Geometry check sheet. Reference: the model listing, model coordinates, mm. A direction names the side the tool comes from. Coordinates: 2 decimals unless noted, no trailing zeros. Loops run counter-clockwise (first coordinate to the right, second up) from the corner with the lowest first, then second, coordinate; pieces in that order, holes last.
from build123d import *
from build123d.topology import SkipClean

# Parameters (mm, degrees)
BOSS_EXTRUDE1_DEPTH = 10
BOSS_EXTRUDE2_DEPTH = 7.5
BOSS_EXTRUDE3_DEPTH = 5


with BuildPart() as part:
    # Sketch1 → Boss-Extrude1 (new, symmetric)
    with SkipClean():  # the faces are left unmerged after this step: merging them gives an invalid solid
        with BuildSketch(Plane.XY):
            with BuildLine():
                Line((-10, 54.083269132), (-10, 42.848570571))
                ThreePointArc((-10, 42.848570571), (0, 44), (10, 42.848570571))
                Line((10, 42.848570571), (10, 54.083269132))
                Line((10, 54.083269132), (10, 89))
                Line((10, 89), (10, 95.679491924))
                ThreePointArc((10, 95.679491924), (0, 93), (-10, 95.679491924))
                Line((-10, 95.679491924), (-10, 89))
                Line((-10, 89), (-10, 54.083269132))
            make_face()
            with BuildLine():
                ThreePointArc((-42.848570571, -10), (-44, 0), (-42.848570571, 10))
                Line((-42.848570571, 10), (-54.083269132, 10))
                Line((-54.083269132, 10), (-89, 10))
                Line((-89, 10), (-95.679491924, 10))
                ThreePointArc((-95.679491924, 10), (-93.681483474, 5.176380902), (-93, 0))
                ThreePointArc((-93, 0), (-93.681483474, -5.176380902), (-95.679491924, -10))
                Line((-95.679491924, -10), (-89, -10))
                Line((-89, -10), (-54.083269132, -10))
                Line((-54.083269132, -10), (-42.848570571, -10))
            make_face()
            with BuildLine():
                ThreePointArc((10, -42.848570571), (0, -44), (-10, -42.848570571))
                Line((-10, -42.848570571), (-10, -54.083269132))
                Line((-10, -54.083269132), (-10, -89))
                Line((-10, -89), (-10, -95.679491924))
                ThreePointArc((-10, -95.679491924), (0, -93), (10, -95.679491924))
                Line((10, -95.679491924), (10, -89))
                Line((10, -89), (10, -54.083269132))
                Line((10, -54.083269132), (10, -42.848570571))
            make_face()
            with BuildLine():
                Line((54.083269132, 10), (42.848570571, 10))
                ThreePointArc((42.848570571, 10), (43.71119482, 5.033035608), (44, 0))
                ThreePointArc((44, 0), (43.71119482, -5.033035608), (42.848570571, -10))
                Line((42.848570571, -10), (54.083269132, -10))
                Line((54.083269132, -10), (89, -10))
                Line((89, -10), (95.679491924, -10))
                ThreePointArc((95.679491924, -10), (93, 0), (95.679491924, 10))
                Line((95.679491924, 10), (89, 10))
                Line((89, 10), (54.083269132, 10))
            make_face()
            with BuildLine():
                ThreePointArc((-18.384776311, 131.384776311), (-25.505709112, 107.954328319), (-10, 89))
                Line((-10, 89), (-10, 95.679491924))
                ThreePointArc((-10, 95.679491924), (-10, 130.320508076), (20, 113))
                ThreePointArc((20, 113), (17.320508076, 103), (10, 95.679491924))
                Line((10, 95.679491924), (10, 89))
                ThreePointArc((10, 89), (25.505709112, 107.954328319), (18.384776311, 131.384776311))
                ThreePointArc((18.384776311, 131.384776311), (0, 139), (-18.384776311, 131.384776311))
            make_face()
            with BuildLine():
                Line((-95.679491924, 10), (-89, 10))
                ThreePointArc((-89, 10), (-107.954328319, 25.505709112), (-131.384776311, 18.384776311))
                ThreePointArc((-131.384776311, 18.384776311), (-134.295069945, -14.917104144), (-102.002815768, -23.559752524))
                ThreePointArc((-102.002815768, -23.559752524), (-94.233874983, -17.995348061), (-89, -10))
                Line((-89, -10), (-95.679491924, -10))
                ThreePointArc((-95.679491924, -10), (-133, 0), (-95.679491924, 10))
            make_face()
            with BuildLine():
                ThreePointArc((131.384776311, 18.384776311), (107.954328319, 25.505709112), (89, 10))
                Line((89, 10), (95.679491924, 10))
                ThreePointArc((95.679491924, 10), (118.176380902, 19.318516526), (133, 0))
                ThreePointArc((133, 0), (118.176380902, -19.318516526), (95.679491924, -10))
                Line((95.679491924, -10), (89, -10))
                ThreePointArc((89, -10), (94.233874983, -17.995348061), (102.002815768, -23.559752524))
                ThreePointArc((102.002815768, -23.559752524), (134.295069945, -14.917104144), (131.384776311, 18.384776311))
            make_face()
            with BuildLine():
                Line((-10, -95.679491924), (-10, -89))
                ThreePointArc((-10, -89), (-17.995348061, -94.233874983), (-23.559752524, -102.002815768))
                ThreePointArc((-23.559752524, -102.002815768), (0, -139), (23.559752524, -102.002815768))
                ThreePointArc((23.559752524, -102.002815768), (17.995348061, -94.233874983), (10, -89))
                Line((10, -89), (10, -95.679491924))
                ThreePointArc((10, -95.679491924), (17.320508076, -103), (20, -113))
                ThreePointArc((20, -113), (-10, -130.320508076), (-10, -95.679491924))
            make_face()
        extrude(amount=BOSS_EXTRUDE1_DEPTH, both=True)

    # Sketch1_3 → Boss-Extrude2 (add, symmetric)
    with BuildSketch(Plane.XY):
        with BuildLine():
            Line((-54.083269132, 10), (-42.848570571, 10))
            ThreePointArc((-42.848570571, 10), (-31.112698372, 31.112698372), (-10, 42.848570571))
            Line((-10, 42.848570571), (-10, 54.083269132))
            ThreePointArc((-10, 54.083269132), (-38.890872965, 38.890872965), (-54.083269132, 10))
        make_face()
        with BuildLine():
            Line((10, 54.083269132), (10, 42.848570571))
            ThreePointArc((10, 42.848570571), (31.112698372, 31.112698372), (42.848570571, 10))
            Line((42.848570571, 10), (54.083269132, 10))
            ThreePointArc((54.083269132, 10), (38.890872965, 38.890872965), (10, 54.083269132))
        make_face()
        with BuildLine():
            ThreePointArc((42.848570571, -10), (31.112698372, -31.112698372), (10, -42.848570571))
            Line((10, -42.848570571), (10, -54.083269132))
            ThreePointArc((10, -54.083269132), (38.890872965, -38.890872965), (54.083269132, -10))
            Line((54.083269132, -10), (42.848570571, -10))
        make_face()
        with BuildLine():
            ThreePointArc((-10, -42.848570571), (-31.112698372, -31.112698372), (-42.848570571, -10))
            Line((-42.848570571, -10), (-54.083269132, -10))
            ThreePointArc((-54.083269132, -10), (-38.890872965, -38.890872965), (-10, -54.083269132))
            Line((-10, -54.083269132), (-10, -42.848570571))
        make_face()
    extrude(amount=BOSS_EXTRUDE2_DEPTH, both=True)

    # Sketch1_4 → Boss-Extrude3 (add, symmetric)
    with BuildSketch(Plane.XY):
        with BuildLine():
            Line((-89, 10), (-54.083269132, 10))
            ThreePointArc((-54.083269132, 10), (-38.890872965, 38.890872965), (-10, 54.083269132))
            Line((-10, 54.083269132), (-10, 89))
            ThreePointArc((-10, 89), (-25.505709112, 107.954328319), (-18.384776311, 131.384776311))
            Line((-18.384776311, 131.384776311), (-131.384776311, 18.384776311))
            ThreePointArc((-131.384776311, 18.384776311), (-107.954328319, 25.505709112), (-89, 10))
        make_face()
        with BuildLine():
            Line((10, 89), (10, 54.083269132))
            ThreePointArc((10, 54.083269132), (38.890872965, 38.890872965), (54.083269132, 10))
            Line((54.083269132, 10), (89, 10))
            ThreePointArc((89, 10), (107.954328319, 25.505709112), (131.384776311, 18.384776311))
            Line((131.384776311, 18.384776311), (18.384776311, 131.384776311))
            ThreePointArc((18.384776311, 131.384776311), (25.505709112, 107.954328319), (10, 89))
        make_face()
        with BuildLine():
            ThreePointArc((-10, -54.083269132), (-38.890872965, -38.890872965), (-54.083269132, -10))
            Line((-54.083269132, -10), (-89, -10))
            ThreePointArc((-89, -10), (-94.233874983, -17.995348061), (-102.002815768, -23.559752524))
            ThreePointArc((-102.002815768, -23.559752524), (-74.773631801, -21.15717706), (-52.359428182, -36.803400392))
            ThreePointArc((-52.359428182, -36.803400392), (-45.254833996, -45.254833996), (-36.803400392, -52.359428182))
            ThreePointArc((-36.803400392, -52.359428182), (-21.15717706, -74.773631801), (-23.559752524, -102.002815768))
            ThreePointArc((-23.559752524, -102.002815768), (-17.995348061, -94.233874983), (-10, -89))
            Line((-10, -89), (-10, -54.083269132))
        make_face()
        with BuildLine():
            ThreePointArc((54.083269132, -10), (38.890872965, -38.890872965), (10, -54.083269132))
            Line((10, -54.083269132), (10, -89))
            ThreePointArc((10, -89), (17.995348061, -94.233874983), (23.559752524, -102.002815768))
            ThreePointArc((23.559752524, -102.002815768), (21.15717706, -74.773631801), (36.803400392, -52.359428182))
            ThreePointArc((36.803400392, -52.359428182), (45.254833996, -45.254833996), (52.359428182, -36.803400392))
            ThreePointArc((52.359428182, -36.803400392), (74.773631801, -21.15717706), (102.002815768, -23.559752524))
            ThreePointArc((102.002815768, -23.559752524), (94.233874983, -17.995348061), (89, -10))
            Line((89, -10), (54.083269132, -10))
        make_face()
    extrude(amount=BOSS_EXTRUDE3_DEPTH, both=True)


solid = part.part
(1) Sectioned sample at D-D on y = -81. Record the cut outline in (x, z).
Findings:
outline: (-20.01, -5) - (-10, -5) - (-10, -10) - (10, -10) - (10, -5) - (20.01, -5) - (20.01, 5) - (10, 5) - (10, 10) - (-10, 10) - (-10, 5) - (-20.01, 5) - close
(2) Scan lines: L1, parallel to X at y = -3, z = -4.25; L2, parallel to Y at x = 13, z = -3.75; L3, parallel to X at y = 113, z = 7.75. Record each from-to range of solid material in increasing order.
Findings:
L1: x = -138.83 to -132.77, -93.23 to -43.9, 43.9 to 93.23, 132.77 to 138.83
L2: y = -135.52 to -128.2, -97.8 to -42.04, 42.04 to 97.8, 128.2 to 135.52
L3: x = -26 to -20, 20 to 26
(3) Sectioned sample at A-A on x = 0. Record the cut outline in (y, z), and give its area (3 significant figures).
Findings:
outline: (-139, -10) - (-133, -10) - (-133, 10) - (-139, 10) - close; (-93, -10) - (-44, -10) - (-44, 10) - (-93, 10) - close; (44, -10) - (93, -10) - (93, 10) - (44, 10) - close; (133, -10) - (139, -10) - (139, 10) - (133, 10) - close
area: 2,200 mm2
(4) Draft check along Y on faces 4 (the flat face through (75.68, 74.09, -0.07)), 5 (the flat face through (0, -87, 10)), 6 (the flat face through (34, -32, -7.5)). Enter one of: +Y half, -Y half, draft (parallel to the pull), parting line (faces both ways), or undercut.
Findings:
face 4: +Y half
face 5: draft
face 6: undercut
(5) Gauge pin test, flat ends, axial feed: pin 1 Ø2.5 at (y, z) = (56, -8) entering from -X; pin 2 Ø22 at (x, y) = (42, 27) entering from -Z; pin 3 Ø8 at (y, z) = (55, 1) entering from -X. Record the tip position at first contact, or that the pin passes through.
Findings:
pin 1: stops at x = -10
pin 2: stops at z = -7.5
pin 3: stops at x = -98.77
(6) Sectioned sample at B-B on y = 33.5. Record the cut outline in (x, z), and give its area (3 significant figures).
Findings:
outline: (-116.27, -5) - (-43.62, -5) - (-43.62, -7.5) - (-28.53, -7.5) - (-28.53, 7.5) - (-43.62, 7.5) - (-43.62, 5) - (-116.27, 5) - close; (28.53, -7.5) - (43.62, -7.5) - (43.62, -5) - (116.27, -5) - (116.27, 5) - (43.62, 5) - (43.62, 7.5) - (28.53, 7.5) - close
area: 1,910 mm2
(7) Sectioned sample at C-C on x = -113. Record the cut outline in (y, z), and give its area (3 significant figures).
Findings:
outline: (-26, -10) - (-20, -10) - (-20, 10) - (-26, 10) - close; (20, -10) - (26, -10) - (26, -5) - (36.77, -5) - (36.77, 5) - (26, 5) - (26, 10) - (20, 10) - close
area: 348 mm2
(8) Access from +Z, -Z, +X, -X, +Y, -Y to the whole of each face (thin tool, end or side, straight path). Record for faces 1 (the flat face through (-92, 0, -10)), 2 (the cylindrical face through (-38.56, 39.22, -6.27)), 3 (the flat face through (-43, -46, 5)).
Findings:
face 1: -Z, +X, -X, +Y, -Y
face 2: -Z
face 3: +Z
